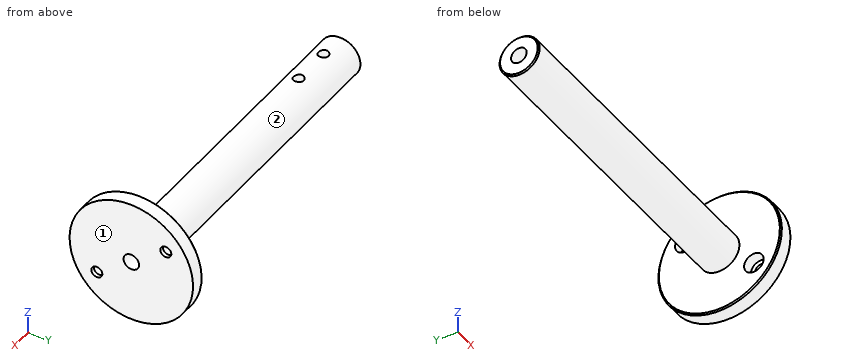
from build123d import *

# Parameters (mm, degrees)
CHANFREIN1_SIZE                                    = 0.5
CHAMBRAGE_POUR_VIS_T_TE_HEXAGONALE_M41_D           = 4.5
CHAMBRAGE_POUR_VIS_T_TE_HEXAGONALE_M41_CBORE_D     = 8
CHAMBRAGE_POUR_VIS_T_TE_HEXAGONALE_M41_CBORE_DEPTH = 4.4
TROU_TARAUD_M51_D                                  = 4.2
TROU_TARAUD_M51_DEPTH                              = 14
TROU_TARAUD_M51_TIP                                = 1.2618073
TROU_TARAUD_M51_ON_FACE_2_D                        = 4.2
TROU_TARAUD_M51_ON_FACE_2_DEPTH                    = 14
TROU_TARAUD_M51_ON_FACE_2_TIP                      = 1.2618073


with BuildPart() as part:
    # Esquisse1 → Révolution1 (revolve)
    with BuildSketch(Plane.XY, mode=Mode.PRIVATE) as r_volution1_sk:
        Polygon((0, 8.175), (129, 8.175), (129, 25.175), (135, 25.175), (135, 3.175), (0, 3.175), align=None)
    revolve(r_volution1_sk.sketch.rotate(Axis((0, 0, 0), (1, 0, 0)), 90), axis=Axis((0, 0, 0), (1, 0, 0)))

    # Chanfrein1
    chanfrein1_edges = [part.edges().sort_by_distance(p)[0] for p in [
        (129, 0, -25.175),
        (0, 0, -8.175),
    ]]
    chamfer(chanfrein1_edges, length=CHANFREIN1_SIZE)

    # Chambrage pour vis à tête hexagonale M41 (through all)
    with Locations(Plane.ZY.offset(-129)):
        with Locations((-10.409398768, -14.067495061), (10.409398768, 14.067495061)):
            CounterBoreHole(CHAMBRAGE_POUR_VIS_T_TE_HEXAGONALE_M41_D / 2, CHAMBRAGE_POUR_VIS_T_TE_HEXAGONALE_M41_CBORE_D / 2, CHAMBRAGE_POUR_VIS_T_TE_HEXAGONALE_M41_CBORE_DEPTH)

    # Trou taraudé M51
    with Locations(Plane(origin=(11.080716358, -0.227251989, 8.171840768), x_dir=(0, 0.999613549573, 0.027798408415), z_dir=(0, -0.027798408415, 0.999613549573))):
        with Locations((0, 0)):
            Hole(TROU_TARAUD_M51_D / 2, depth=TROU_TARAUD_M51_DEPTH)
            with Locations((0, 0, -(TROU_TARAUD_M51_DEPTH + TROU_TARAUD_M51_TIP / 2))):  # 118° drill point
                Cone(0, TROU_TARAUD_M51_D / 2, TROU_TARAUD_M51_TIP, mode=Mode.SUBTRACT)

    # Trou taraudé M51 on face 2
    with Locations(Plane(origin=(27.080716358, -0.227251989, 8.171840768), x_dir=(0, 0.99961356127, 0.027797987799), z_dir=(0, -0.027797987799, 0.99961356127))):
        with Locations((0, 0)):
            Hole(TROU_TARAUD_M51_ON_FACE_2_D / 2, depth=TROU_TARAUD_M51_ON_FACE_2_DEPTH)
            with Locations((0, 0, -(TROU_TARAUD_M51_ON_FACE_2_DEPTH + TROU_TARAUD_M51_ON_FACE_2_TIP / 2))):  # 118° drill point
                Cone(0, TROU_TARAUD_M51_ON_FACE_2_D / 2, TROU_TARAUD_M51_ON_FACE_2_TIP, mode=Mode.SUBTRACT)


solid = part.part
Model file for the job. Use its own axes, mm. Face numbers are marked on the shaded views. A direction names the side the tool comes from. Give positions to 0.01 mm unless a question says otherwise; leave off trailing zeros. Loops run counter-clockwise (first coordinate to the right, second up) from the corner with the lowest first, then second, coordinate; pieces in that order, holes last.
Item 1: Slice it at B-B (x = 86). Write the cut outline in (y, z) (3 decimals), plus the area to 3 significant figures.
Check values:
outline: circle Ø16.35 at (0, 0); hole circle Ø6.35 at (0, 0)
area: 178 mm2
Item 2: Slice it at A-A (z = 0). Write the cut outline in (x, y) (3 decimals).
Check values:
outline: (0, -7.675) - (0.5, -8.175) - (129, -8.175) - (129, -24.675) - (129.5, -25.175) - (135, -25.175) - (135, -3.175) - (0, -3.175) - close; (0, 3.175) - (135, 3.175) - (135, 25.175) - (129.5, 25.175) - (129, 24.675) - (129, 8.175) - (0.5, 8.175) - (0, 7.675) - close
Item 3: Drill centre lines: line 1 along X through (y, z) = (-13, 11.5); line 2 along Y through (x, z) = (10.5, -1.5); line 3 along X through (y, z) = (13.5, 7). Where is each one in solid material? Low to high.
Check values:
line 1: x = 129 to 135
line 2: y = -8.04 to -2.8, 2.8 to 8.04
line 3: x = 133.4 to 135
Item 4: Which spindle directions (+Z, -Z, +X, -X, +Y, -Y) get a long thin tool onto all of the face, cutting with end or side? Do the marked faces 1 and 2. Say none if no direction does.
Check values:
face 1: +Z, -Z, +X, +Y, -Y
face 2: -X
Item 5: Drop flat-ended pins along their axis: P1, Ø6, axis at y = -17.5, z = 12.5, coming from the -X side; P2, Ø12, axis at x = 26, y = 9, coming from the +Z side; P3, Ø8, axis at x = 53, z = 1, coming from the -Y side (3 decimals). Give the stop position or say it passes through.
Check values:
P1: stops at x = 129
P2: stops at z = 7.6
P3: stops at y = -8.175
